Geometry: final body of the model. Coordinates: model frame, mm. A direction names the side the tool comes from. Give positions to 0.01 mm unless a question says otherwise; leave off trailing zeros. Order: outer loops, then holes, each group sorted by start corner. A loop starts at its lowest first (then second) coordinate and runs counter-clockwise, first axis right, second up. Notation, with made-up numbers: (81.25, -28) -> (113.25, -28) arc R26 ccw to (113.25, -12) -> close; hole circle Ø1 at (86, 37). An arc over 180 degrees is marked (long way). One line per item, written item: value. Start each with the question number.
```python
from build123d import *

# Parameters (mm, degrees)
SKETCH1_R           = 11.1125
SKETCH1_R_2         = 4.7625
BOSS_EXTRUDE1_DEPTH = 7.14375
SKETCH2_R           = 9.8425
SKETCH2_R_2         = 6.6675
CUT_EXTRUDE1_DEPTH  = 0.127
SKETCH3_R           = 9.8425
SKETCH3_R_2         = 6.6675
CUT_EXTRUDE3_DEPTH  = 0.127
FILLET1_R           = 0.381


with BuildPart() as part:
    # Sketch1 → Boss-Extrude1 (new body)
    with BuildSketch(Plane(origin=(0, 0, 0), x_dir=(1, 0, 0), z_dir=(0, 1, 0))):
        Circle(SKETCH1_R)
        Circle(SKETCH1_R_2, mode=Mode.SUBTRACT)
    extrude(amount=BOSS_EXTRUDE1_DEPTH)

    # Sketch2 → Cut-Extrude1 (cut)
    with BuildSketch(Plane(origin=(0, 7.14375, 0), x_dir=(1, 0, 0), z_dir=(0, 1, 0))):
        Circle(SKETCH2_R)
        Circle(SKETCH2_R_2, mode=Mode.SUBTRACT)
    extrude(amount=-CUT_EXTRUDE1_DEPTH, mode=Mode.SUBTRACT)

    # Sketch3 → Cut-Extrude3 (cut)
    with BuildSketch(Plane.XZ):
        Circle(SKETCH3_R)
        Circle(SKETCH3_R_2, mode=Mode.SUBTRACT)
    extrude(amount=-CUT_EXTRUDE3_DEPTH, mode=Mode.SUBTRACT)

    # Fillet1
    fillet1_edges = [part.edges().sort_by_distance(p)[0] for p in [
        (-11.1125, 0, 0),
        (-11.1125, 7.14375, 0),
    ]]
    fillet(fillet1_edges, radius=FILLET1_R)


solid = part.part
```
1. Draft query along X for faces 1 (the cylindrical face through (10.6, 3.53, -3.34)), 2 (the flat face through (-2, 7.144, -5)), 3 (the flat face through (-2.33, 0.127, -6.42)). Return one class per face: pulls with the +X half, pulls with the -X half, needs draft (parallel to the pull), parting line crosses it, or undercut.
2. Cut plane A-A, the plane z = 0. Return loops of the section in (x, y).
3. Material intervals for L1, parallel to X at y = 3.75, z = 0; L2, parallel to Y at x = 5.5, z = 6.25, sorted ascending. Write a range as [from, to].
4. Access query for faces 4 (the cylindrical face through (-3.78, 3.52, 2.9)), 5 (the flat face through (-2.33, 7.017, 6.42)). Directions: +Z, -Z, +X, -X, +Y, -Y. A direction counts if a zero-diameter tool reaches every point of the face in a straight line with its end or side. Return the directions, or none.
5. Cut plane C-C, the plane y = 4. Return loops of the section in (x, z) (1 decimal).
6. Pin query (flat end, axial travel): P1, Ø2, axis at y = 3.5, z = -9, coming from the -X side. Return the tip coordinate at first contact, or that it passes through.
7. Cut plane B-B, the plane x = 0. Return loops of the section in (y, z), then the cut area to 3 significant figures.
Answers follow:
1. face 1: parting line crosses it
1. face 2: needs draft
1. face 3: undercut
2. outline: (-11.11, 0.38) arc R0.38 ccw to (-10.73, 0) -> (-9.84, 0) -> (-9.84, 0.13) -> (-6.67, 0.13) -> (-6.67, 0) -> (-4.76, 0) -> (-4.76, 7.14) -> (-6.67, 7.14) -> (-6.67, 7.02) -> (-9.84, 7.02) -> (-9.84, 7.14) -> (-10.73, 7.14) arc R0.38 ccw to (-11.11, 6.76) -> close; (4.76, 0) -> (6.67, 0) -> (6.67, 0.13) -> (9.84, 0.13) -> (9.84, 0) -> (10.73, 0) arc R0.38 ccw to (11.11, 0.38) -> (11.11, 6.76) arc R0.38 ccw to (10.73, 7.14) -> (9.84, 7.14) -> (9.84, 7.02) -> (6.67, 7.02) -> (6.67, 7.14) -> (4.76, 7.14) -> close
3. L1: x = [-11.11, -4.76], [4.76, 11.11]
3. L2: y = [0.13, 7.02]
4. face 4: +Y, -Y
4. face 5: +Y
5. outline: circle Ø22.2 at (0, 0); hole circle Ø9.5 at (0, 0)
6. P1: stops at x = -7.71
7. outline: (0, -10.73) arc R0.38 ccw to (0.38, -11.11) -> (6.76, -11.11) arc R0.38 ccw to (7.14, -10.73) -> (7.14, -9.84) -> (7.02, -9.84) -> (7.02, -6.67) -> (7.14, -6.67) -> (7.14, -4.76) -> (0, -4.76) -> (0, -6.67) -> (0.13, -6.67) -> (0.13, -9.84) -> (0, -9.84) -> close; (0, 4.76) -> (7.14, 4.76) -> (7.14, 6.67) -> (7.02, 6.67) -> (7.02, 9.84) -> (7.14, 9.84) -> (7.14, 10.73) arc R0.38 ccw to (6.76, 11.11) -> (0.38, 11.11) arc R0.38 ccw to (0, 10.73) -> (0, 9.84) -> (0.13, 9.84) -> (0.13, 6.67) -> (0, 6.67) -> close
7. area: 89.0 mm²
